Check sheet for the drawn part. Datum: minimum x, y, z corner. Units: mm. Coordinates: 2 decimals unless noted, no trailing zeros. Write each loop counter-clockwise with the first axis right and the second up, starting at its lowest first coordinate (ties: lowest second). Pieces come first, ordered by that corner, then holes. Notation, with made-up numbers: M -4.5,15.5 L 38.5,15.5 A19 cw 38.5,39.5 Z; hole C 39,67 d1. An arc over 180 degrees is marked long. Answer as CSV lines item,"result". Start each with the question number.
Q1. Sectioned sample at A-A, the plane z = 10. Record the cut outline in (x, y).
Q2. Sectioned sample at D-D, the plane z = 4.25. Record the cut outline in (x, y).
Q3. Sectioned sample at C-C, the plane x = 3.75. Record the cut outline in (y, z), then the cut area to 3 significant figures.
Q4. Thickness scan on line 1 along X through (y, z) = (0.7, 10); line 2 along X through (y, z) = (0.2, 4.25); line 3 along Z through (x, y) = (3.75, 1.25). Record the ranges inside material, lowest first. Write a range as from..to.
Q5. Sectioned sample at B-B, the plane y = 1.3. Record the cut outline in (x, z).
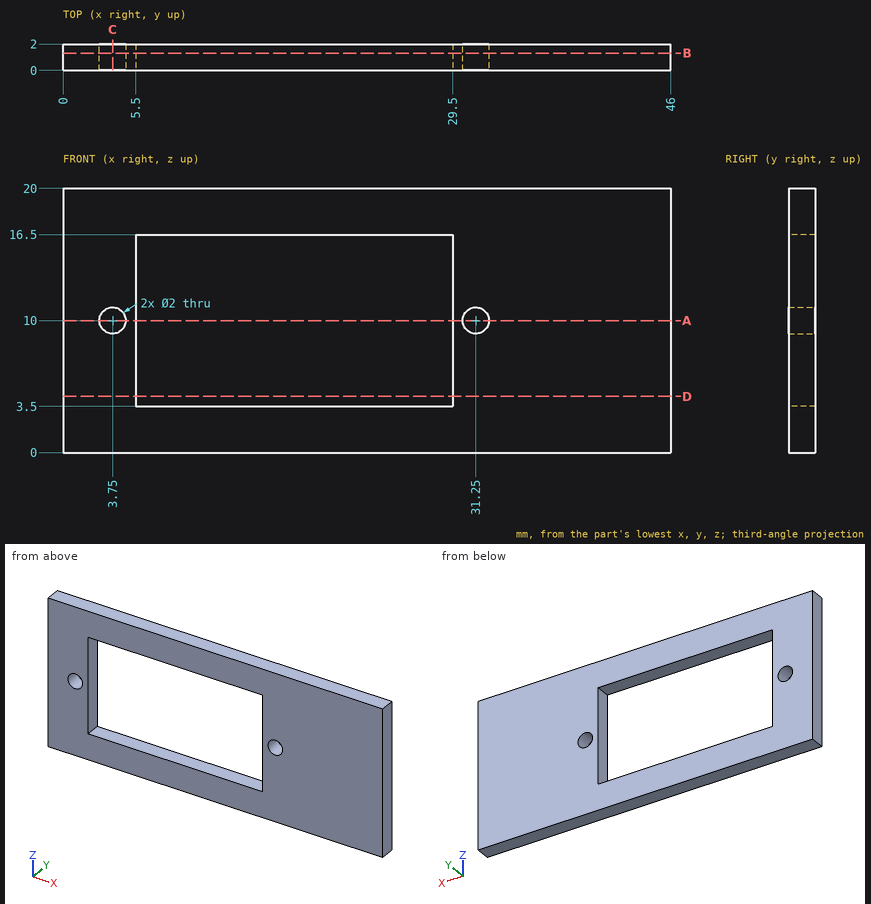
Output:
1,outline,"M 0,0 L 2.75,0 L 2.75,2 L 0,2 Z; M 4.75,0 L 5.5,0 L 5.5,2 L 4.75,2 Z; M 29.5,0 L 30.25,0 L 30.25,2 L 29.5,2 Z; M 32.25,0 L 46,0 L 46,2 L 32.25,2 Z"
2,outline,"M 0,0 L 5.5,0 L 5.5,2 L 0,2 Z; M 29.5,0 L 46,0 L 46,2 L 29.5,2 Z"
3,outline,"M 0,0 L 2,0 L 2,9 L 0,9 Z; M 0,11 L 2,11 L 2,20 L 0,20 Z"
3,area,"36.0 mm^2"
4,line 1,"x = 0..2.75, 4.75..5.5, 29.5..30.25, 32.25..46"
4,line 2,"x = 0..5.5, 29.5..46"
4,line 3,"z = 0..9, 11..20"
5,outline,"M 0,0 L 46,0 L 46,20 L 0,20 Z; hole C 3.75,10 d2; hole M 5.5,3.5 L 29.5,3.5 L 29.5,16.5 L 5.5,16.5 Z; hole C 31.25,10 d2"
